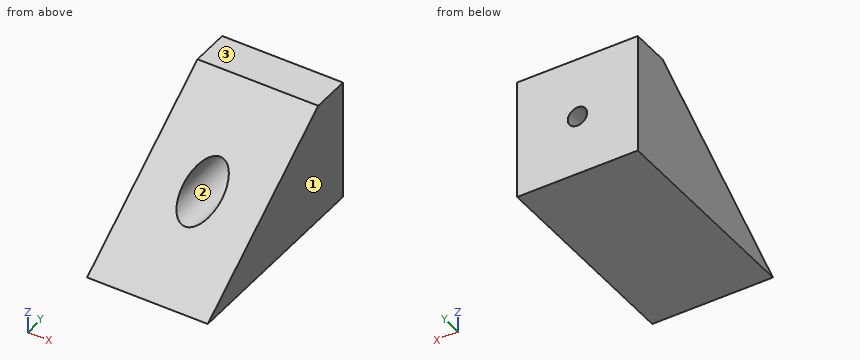
from build123d import *

# Parameters (mm, degrees)
PAD006_DEPTH    = 12.5
SKETCH011_R     = 1
POCKET015_DEPTH = 50
SKETCH_R        = 2
POCKET_DEPTH    = 21.85185


with BuildPart() as part:
    # Sketch010 → Pad006 (new body)
    with BuildSketch(Plane.YZ):
        Polygon((-21.85185, 0), (0, 0), (0, 12.5), (-4, 12.5), align=None)
    extrude(amount=PAD006_DEPTH)

    # Sketch011 → Pocket015 (cut)
    with BuildSketch(Plane.XZ):
        with Locations((6.25, 6.25)):
            Circle(SKETCH011_R)
    extrude(amount=POCKET015_DEPTH, mode=Mode.SUBTRACT)

    # Sketch (on DatumPlane) → Pocket (cut)
    with BuildSketch(Plane.XZ.offset(4)):
        with Locations((6.25, 6.25)):
            Circle(SKETCH_R)
    extrude(amount=POCKET_DEPTH, mode=Mode.SUBTRACT)


solid = part.part
CAD build for the part. Positions are in the model's coordinates, mm. Face numbers are marked on the shaded views. Coordinates: 2 decimals unless noted, no trailing zeros. Order: outer loops, then holes, each group sorted by start corner. A loop starts at its lowest first (then second) coordinate and runs counter-clockwise, first axis right, second up.
Item 1: Pin check, flat tips, straight feed: pin 1 Ø1.5 at (x, z) = (8.5, 2) entering from -Y; pin 2 Ø1.2 at (x, z) = (6.25, 6.25) entering from +Y; pin 3 Ø2 at (x, z) = (5.5, 9) entering from -Y; pin 4 Ø4.5 at (x, z) = (6, 6) entering from -Y. Stop position of each tip, or through.
Check sheet entries:
pin 1: stops at y = -20.07
pin 2: passes through
pin 3: stops at y = -10.4
pin 4: stops at y = -16.5
Item 2: Band-saw the part on A-A on z = 6.25. List the corners of the cut face in (x, y), plus the area to 3 significant figures.
Check sheet entries:
outline: (0, -12.93) - (4.25, -12.93) - (4.25, -4) - (5.25, -4) - (5.25, 0) - (0, 0) - close; (7.25, -4) - (8.25, -4) - (8.25, -12.93) - (12.5, -12.93) - (12.5, 0) - (7.25, 0) - close
area: 118 mm2
Item 3: Drill centre lines: L1, parallel to X at y = -12.5, z = 6.25; L2, parallel to X at y = -3.1, z = 6.25. Where is each one in solid material? Low to high.
Check sheet entries:
L1: x = 0 to 4.25, 8.25 to 12.5
L2: x = 0 to 5.25, 7.25 to 12.5
Item 4: Band-saw the part on D-D on z = 7.5. List the corners of the cut face in (x, y), plus the area to 3 significant figures.
Check sheet entries:
outline: (0, -11.14) - (4.69, -11.14) - (4.69, -4) - (7.81, -4) - (7.81, -11.14) - (12.5, -11.14) - (12.5, 0) - (0, 0) - close
area: 117 mm2
Item 5: Band-saw the part on B-B on x = 6.25. List the corners of the cut face in (y, z).
Check sheet entries:
outline: (-21.85, 0) - (0, 0) - (0, 5.25) - (-4, 5.25) - (-4, 4.25) - (-15.78, 4.25) - close; (-10.07, 8.25) - (-4, 8.25) - (-4, 7.25) - (0, 7.25) - (0, 12.5) - (-4, 12.5) - close
Item 6: Two-plate mould, pull along Z, no slides. Class the marked faces 1, 2 and 3: +Z half, -Z half, draft (parallel to the pull), parting line (faces both ways), or undercut.
Check sheet entries:
face 1: draft
face 2: undercut
face 3: +Z half
Item 7: Band-saw the part on C-C on y = -9.75. List the corners of the cut face in (x, z).
Check sheet entries:
outline: (0, 0) - (12.5, 0) - (12.5, 8.47) - (0, 8.47) - close; hole circle Ø4 at (6.25, 6.25)
